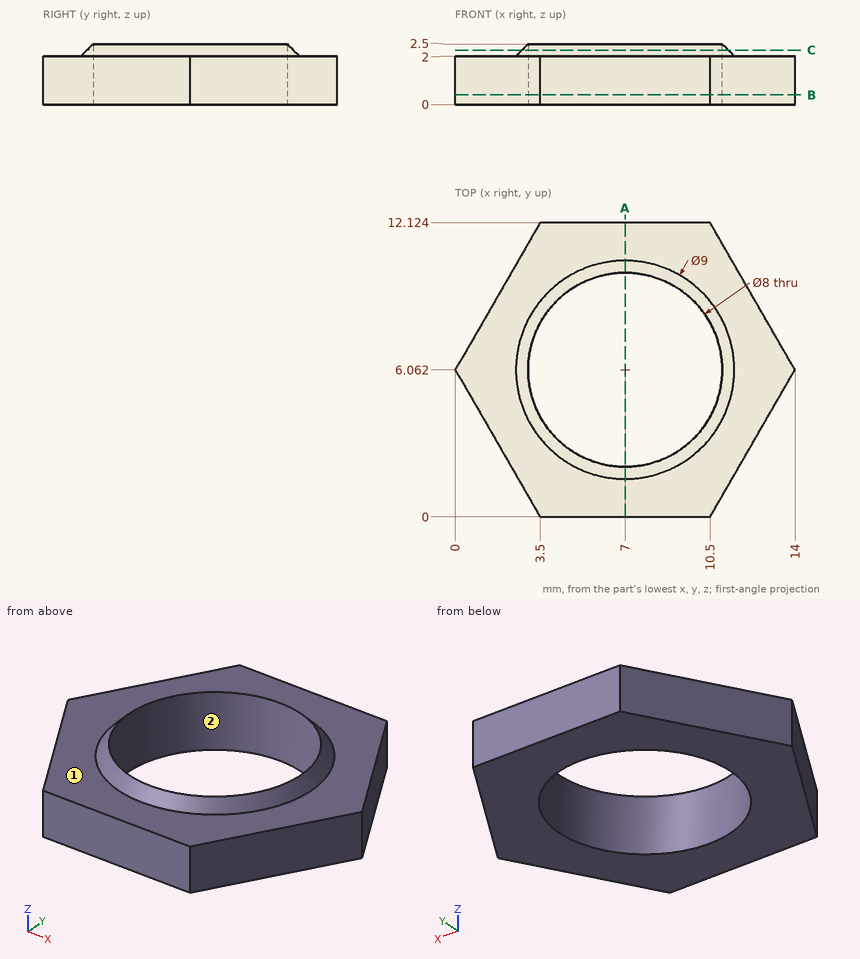
Design review of the part shown in the three views and the two pictorial views. Dimensions are in mm from the part's minimum x, y and z. A direction names the side the tool comes from. Coordinates: 2 decimals unless noted, no trailing zeros. Loops run counter-clockwise (first coordinate to the right, second up) from the corner with the lowest first, then second, coordinate; pieces in that order, holes last.
(1) Insertion check: P1, Ø1, axis at y = 4, z = 1.5, coming from the -X side; P2, Ø1, axis at x = 2.5, y = 8, coming from the -Z side. Each pin has a flat end and moves straight along its axis. Give the tip position at first contact, or say it passes through.
Determined:
P1: stops at x = 0.9
P2: stops at z = 0
(2) Tool access review of the marked faces 1 and 2: name each direction out of +Z, -Z, +X, -X, +Y, -Y from which nothing blocks a thin tool from reaching the whole face with its end or side.
Determined:
face 1: +Z
face 2: +Z, -Z
(3) Wall thickness on L1, parallel to Y at x = 7, z = 0.5 (1 decimal); L2, parallel to Z at x = 4, y = 10; L3, parallel to X at y = 3.75, z = 1.9 (1 decimal): over which ranges is each line inside the solid? List them lowest first.
Determined:
L1: y = 0 to 2.1, 10.1 to 12.1
L2: z = 0 to 2
L3: x = 1.3 to 3.7, 10.3 to 12.7
(4) Consider section A-A, the plane x = 7. Give the boundary of the cut face in (y, z) (1 decimal).
Determined:
outline: (0, 0) - (2.1, 0) - (2.1, 2.5) - (1.6, 2) - (0, 2) - close; (10.1, 0) - (12.1, 0) - (12.1, 2) - (10.6, 2) - (10.1, 2.5) - close
(5) Consider section C-C, the plane z = 2.25. Give the boundary of the cut face in (x, y).
Determined:
outline: circle Ø8.5 at (7, 6.06); hole circle Ø8 at (7, 6.06)
(6) Consider section B-B, the plane z = 0.4. Give the boundary of the cut face in (x, y) (1 decimal).
Determined:
outline: (0, 6.1) - (3.5, 0) - (10.5, 0) - (14, 6.1) - (10.5, 12.1) - (3.5, 12.1) - close; hole circle Ø8 at (7, 6.1)
